Read the model definition and answer for the solid it produces. Units are mm, in the model's axes. Give positions to 0.01 mm unless a question says otherwise; leave off trailing zeros. Order: outer loops, then holes, each group sorted by start corner. A loop starts at its lowest first (then second) coordinate and runs counter-clockwise, first axis right, second up. Notation, with made-up numbers: (32, 32.25) - (61, 32.25) arc R11 cw to (61, 37.25) - close; hole circle Ø5 at (-1, 25). An arc over 180 degrees is marked (long way). Return JSON: item names as keys, results as strings.
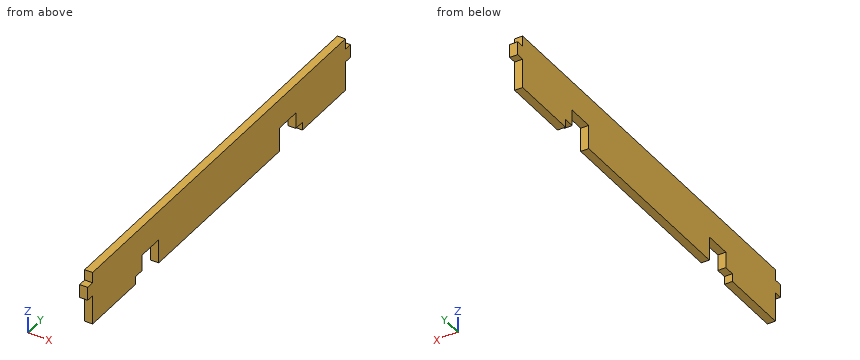
Autodesk Inventor part; units mm, degrees
ref_plane "YZ Plane" through (0, 0, 0) normal (1, 0, 0) x (0, 1, 0)
ref_plane "XZ Plane" through (0, 0, 0) normal (0, 1, 0) x (-1, 0, 0)
ref_plane "XY Plane" through (0, 0, 0) normal (0, 0, 1) x (1, 0, 0)
sketch "Sketch1" plane through (0, 0, 0) normal (1, 0, 0) x (0, 1, 0)
  line L0 (0, 11) -> (-3, 11)
  line L1 (-3, 11) -> (-3, 16)
  line L2 (-3, 16) -> (0, 16)
  line L3 (0, 20) -> (0, 16)
  line L4 (0, 11) -> (0, 0)
  line L5 (153, 16) -> (156, 16)
  line L6 (156, 16) -> (156, 11)
  line L7 (156, 11) -> (153, 11)
  line L8 (153, 0) -> (153, 11)
  line L9 (153, 16) -> (153, 20)
  line L10 (30, 3) -> (30, 9)
  line L11 (30, 9) -> (40, 9)
  line L12 (40, 9) -> (40, 0)
  line L13 (113, 0) -> (113, 9)
  line L14 (113, 9) -> (123, 9)
  line L15 (123, 9) -> (123, 3)
  line L16 (127, 0) -> (153, 0)
  line L17 (0, 0) -> (26, 0)
  line L18 (40, 0) -> (113, 0)
  line L19 (153, 20) -> (0, 20)
  line L20 (30, 3) -> (26, 3)
  line L21 (26, 3) -> (26, 0)
  line L22 (123, 3) -> (127, 3)
  line L23 (127, 3) -> (127, 0)
  dimension "d0" = 20
  dimension "d1" = 153
  dimension "d2" = 5
  dimension "d3" = 3
  dimension "d5" = 3
  dimension "d6" = 5
  dimension "d7" = 10
  dimension "d9" = 30
  dimension "d11" = 10
  dimension "d12" = 30
  dimension "d21" = 11
  dimension "d25" = 4
  dimension "d26" = 3
  dimension "d28" = 4
  dimension "d30" = 9
  dimension "d31" = 9
  dimension "d32" = 9
  dimension "d33" = 20
  dimension "d34" = 3
  dimension "d35" = 26
extrude "Extrusion2" add sketch "Sketch1" along normal blind 3
properties part number "MainPanelWall3"
Q1. A cutting plane is placed at B-B (x = 2.5). Write down the section's boundary in (y, z), and give its area (3 significant figures).
Values:
{"outline": "(-3, 11) - (0, 11) - (0, 0) - (26, 0) - (26, 3) - (30, 3) - (30, 9) - (40, 9) - (40, 0) - (113, 0) - (113, 9) - (123, 9) - (123, 3) - (127, 3) - (127, 0) - (153, 0) - (153, 11) - (156, 11) - (156, 16) - (153, 16) - (153, 20) - (0, 20) - (0, 16) - (-3, 16) - close", "area": "2,890 mm²"}
Q2. Given pin 1 (1.5 mm diameter, centred on x = 1, z = 5, fed in from +Y); pin 2 (5 mm diameter, centred on y = 53, z = 3, fed in from -X); pin 3 (0.9 mm diameter, centred on x = 2, y = -2, fed in from -Z); pin 4 (1.5 mm diameter, centred on x = 1, y = -1, fed in from +Z), each flat-ended and moving along its own axis, determine where each tip first touches the part or whether it passes through.
Values:
{"pin 1": "stops at y = 153", "pin 2": "stops at x = 0", "pin 3": "stops at z = 11", "pin 4": "stops at z = 16"}
Q3. A cutting plane is placed at A-A (z = 4.5). Write down the section's boundary in (x, y), and give its area (3 significant figures).
Values:
{"outline": "(0, 0) - (3, 0) - (3, 30) - (0, 30) - close; (0, 40) - (3, 40) - (3, 113) - (0, 113) - close; (0, 123) - (3, 123) - (3, 153) - (0, 153) - close", "area": "399 mm²"}
Q4. Consider L1, parallel to Y at x = 0.35, z = 8; L2, parallel to Y at x = 2.55, z = 18.5; L3, parallel to Z at x = 1.85, y = 117. Determine where each line is inside the solid, lowest interval first.
Values:
{"L1": "y = 0 to 30, 40 to 113, 123 to 153", "L2": "y = 0 to 153", "L3": "z = 9 to 20"}
Q5. A cutting plane is placed at C-C (y = 34). Write down the section's boundary in (x, z).
Values:
{"outline": "(0, 9) - (3, 9) - (3, 20) - (0, 20) - close"}
Q6. A cutting plane is placed at D-D (z = 18.5). Write down the section's boundary in (x, y), and give its area (3 significant figures).
Values:
{"outline": "(0, 0) - (3, 0) - (3, 153) - (0, 153) - close", "area": "459 mm²"}
